Design review of the part built by this model. Coordinates are the model's own, in mm. A direction names the side the tool comes from. Coordinates: 2 decimals unless noted, no trailing zeros. Order: outer loops, then holes, each group sorted by start corner. A loop starts at its lowest first (then second) coordinate and runs counter-clockwise, first axis right, second up. Notation, with made-up numbers: M 55,-16 L 68,-16 A22 ccw 68,21 Z; hole C -31.5,19.25 d7. An arc over 180 degrees is marked long. Answer as a JSON object with one key per item and string values.
from build123d import *

# Parameters (mm, degrees)
F0_W     = 300
F0_H     = 1000
F1_DEPTH = 19.05
F2_W     = 50.8
F2_H     = 38.1
F3_DEPTH = 19.05
F4_R     = 50


# Not quite as in the source:
# - a length typed as a fraction of an inch, garbled in the dataset ("3 / 203.2 mm" for 3/8 in), is restored


with BuildPart() as f1:
    # F0 (on Top) → F1 (new body)
    with BuildSketch(Plane.XY):
        with Locations((150, 500)):
            Rectangle(F0_W, F0_H)
    extrude(amount=F1_DEPTH)

    # F2 (on face) → F3 (cut, through all)
    with BuildSketch(Plane.XY.offset(19.05)):
        with Locations((50.8, 44.45)):
            Rectangle(F2_W, F2_H)
        with Locations((50.8, 955.55)):
            Rectangle(F2_W, F2_H)
    extrude(amount=-F3_DEPTH, mode=Mode.SUBTRACT)

    # F4
    f4_edges = [f1.edges().sort_by_distance(p)[0] for p in [
        (300, 0, 9.525),
        (300, 1000, 9.525),
    ]]
    fillet(f4_edges, radius=F4_R)


solid = f1.part
1) To check wall thickness, follow L1, parallel to Y at x = 34.5, z = 11.75. State the ranges of the line that lie inside material, in increasing order.
Taken from the geometry:
{"L1": "y = 0 to 25.4, 63.5 to 936.5, 974.6 to 1000"}
2) Add section A-A (z = 14.5). State the section outline as (x, y) points.
Taken from the geometry:
{"outline": "M 0,0 L 250,0 A50 ccw 300,50 L 300,950 A50 ccw 250,1000 L 0,1000 Z; hole M 25.4,25.4 L 76.2,25.4 L 76.2,63.5 L 25.4,63.5 Z; hole M 25.4,936.5 L 76.2,936.5 L 76.2,974.6 L 25.4,974.6 Z"}
3) Mouldability with a two-part tool opening along X and no side actions: class faces 1 (the flat face through (123, 1000, 9)), 2 (the flat face through (76.2, 955, 10)), 3 (the cylindrical face through (284.964, 985.742, 9.658)) as released by +X, released by -X, zero draft, split by the parting line, or undercut.
Taken from the geometry:
{"face 1": "zero draft", "face 2": "undercut", "face 3": "released by +X"}
4) Tool access review of faces 4 (the flat face through (148, 507, 19.05)), 5 (the flat face through (76.2, 44, 10)): name each direction out of +Z, -Z, +X, -X, +Y, -Y from which nothing blocks a thin tool from reaching the whole face with its end or side.
Taken from the geometry:
{"face 4": "+Z, +X, -X, +Y, -Y", "face 5": "+Z, -Z"}
5) Insertion check: pin 1 Ø5.5 at (y, z) = (958.5, 7) entering from +X; pin 2 Ø2 at (x, y) = (34, 836.5) entering from -Z. Each pin has a flat end and moves straight along its axis. Give the tip position at first contact, or say it passes through.
Taken from the geometry:
{"pin 1": "stops at x = 299.67", "pin 2": "stops at z = 0"}
6) Add section B-B (x = 54). State the section outline as (y, z) points.
Taken from the geometry:
{"outline": "M 0,0 L 25.4,0 L 25.4,19.05 L 0,19.05 Z; M 63.5,0 L 936.5,0 L 936.5,19.05 L 63.5,19.05 Z; M 974.6,0 L 1000,0 L 1000,19.05 L 974.6,19.05 Z"}
